from build123d import *

# Parameters (mm, degrees)
SKETCH_1_W          = 8
SKETCH_1_H          = 8
EXTRUDE_1_DEPTH     = 100
SKETCH_2_R          = 2
CUT_EXTRUDE_1_DEPTH = 104


with BuildPart() as part:
    # 草图1 → 凸台-拉伸1 (new body)
    with BuildSketch(Plane.XY):
        Polygon((-1, 5.896797153), (-1, 9), (9, 9), (9, -1), (-1, -1), align=None)
        with Locations((4, 4)):
            Rectangle(SKETCH_1_W, SKETCH_1_H, mode=Mode.SUBTRACT)
    extrude(amount=EXTRUDE_1_DEPTH)

    # 草图2 → 切除-拉伸1 (cut)
    with BuildSketch(Plane(origin=(0, 9, 0), x_dir=(1, 0, 0), z_dir=(0, 1, 0))):
        with Locations(Location((4, -90, 0), (0, 0, 270))):
            Circle(SKETCH_2_R)
        with Locations(Location((4, -10, 0), (0, 0, 270))):
            Circle(SKETCH_2_R)
    extrude(amount=-CUT_EXTRUDE_1_DEPTH, mode=Mode.SUBTRACT)


solid = part.part
Design review of the part built by this model. Coordinates are the model's own, in mm. A direction names the side the tool comes from. Coordinates: 2 decimals unless noted, no trailing zeros. Order: outer loops, then holes, each group sorted by start corner. A loop starts at its lowest first (then second) coordinate and runs counter-clockwise, first axis right, second up. Notation, with made-up numbers: (64.5, 69.25) - (87.5, 69.25) arc R18 cw to (87.5, 94.25) - close; hole circle Ø3 at (20.25, 82). An arc over 180 degrees is marked (long way). Put each result on its own line as item: value.
1) Wall thickness on L1, parallel to Y at x = 7, z = 45.5; L2, parallel to X at y = 8.35, z = 90: over which ranges is each line inside the solid? List them lowest first. Write a range as from..to.
Response values:
L1: y = -1..0, 8..9
L2: x = -1..2, 6..9
2) Take a section at A-A, the plane x = 4. Give the boundary of the cut face in (y, z), and give its area (3 significant figures).
Response values:
outline: (-1, 0) - (0, 0) - (0, 8) - (-1, 8) - close; (-1, 12) - (0, 12) - (0, 88) - (-1, 88) - close; (-1, 92) - (0, 92) - (0, 100) - (-1, 100) - close; (8, 0) - (9, 0) - (9, 8) - (8, 8) - close; (8, 12) - (9, 12) - (9, 88) - (8, 88) - close; (8, 92) - (9, 92) - (9, 100) - (8, 100) - close
area: 184 mm²
3) Tool access review of faces 1 (the face through (4, 8, 49)), 2 (the face through (-1, 4, 49)): name each direction out of +Z, -Z, +X, -X, +Y, -Y from which nothing blocks a thin tool from reaching the whole face with its end or side.
Response values:
face 1: +Z, -Z
face 2: +Z, -Z, -X, +Y, -Y
4) Take a section at B-B, the plane z = 83. Give the boundary of the cut face in (x, y), and give its area (3 significant figures).
Response values:
outline: (-1, -1) - (9, -1) - (9, 9) - (-1, 9) - close; hole (0, 0) - (8, 0) - (8, 8) - (0, 8) - close
area: 36.0 mm²
5) Take a section at D-D, the plane z = 10. Give the boundary of the cut face in (x, y).
Response values:
outline: (-1, -1) - (2, -1) - (2, 0) - (0, 0) - (0, 8) - (2, 8) - (2, 9) - (-1, 9) - close; (6, -1) - (9, -1) - (9, 9) - (6, 9) - (6, 8) - (8, 8) - (8, 0) - (6, 0) - close
6) The part is to be moulded in two halves that separate along Z. For faces 3 (the face through (8.5, 4.1, 100)), 4 (the face through (0, 4, 49)), 5 (the face through (4.601, 8.507, 91.908)), 6 (the face through (2.048, -0.493, 9.566)), say which applies: released by +Z, released by -Z, zero draft, split by the parting line, or undercut.
Response values:
face 3: released by +Z
face 4: zero draft
face 5: undercut
face 6: undercut
7) Take a section at C-C, the plane y = 1.5. Give the boundary of the cut face in (x, z).
Response values:
outline: (-1, 0) - (0, 0) - (0, 100) - (-1, 100) - close; (8, 0) - (9, 0) - (9, 100) - (8, 100) - close
